The figure shows three views and two pictorial views of one solid part (mm, origin at its lowest corner). Answer the questions. Give positions to 0.01 mm unless a question says otherwise; leave off trailing zeros. Write each loop counter-clockwise with the first axis right and the second up, starting at its lowest first coordinate (ties: lowest second). Pieces come first, ordered by that corner, then holes. Notation, with made-up numbers: (-3.5, 88.5) -> (26.5, 88.5) arc R17 cw to (26.5, 101.5) -> close; hole circle Ø2 at (-24.5, 12.5). An arc over 180 degrees is marked (long way). Write each question's results on one line, items separated by ' | '. Start each with the question number.
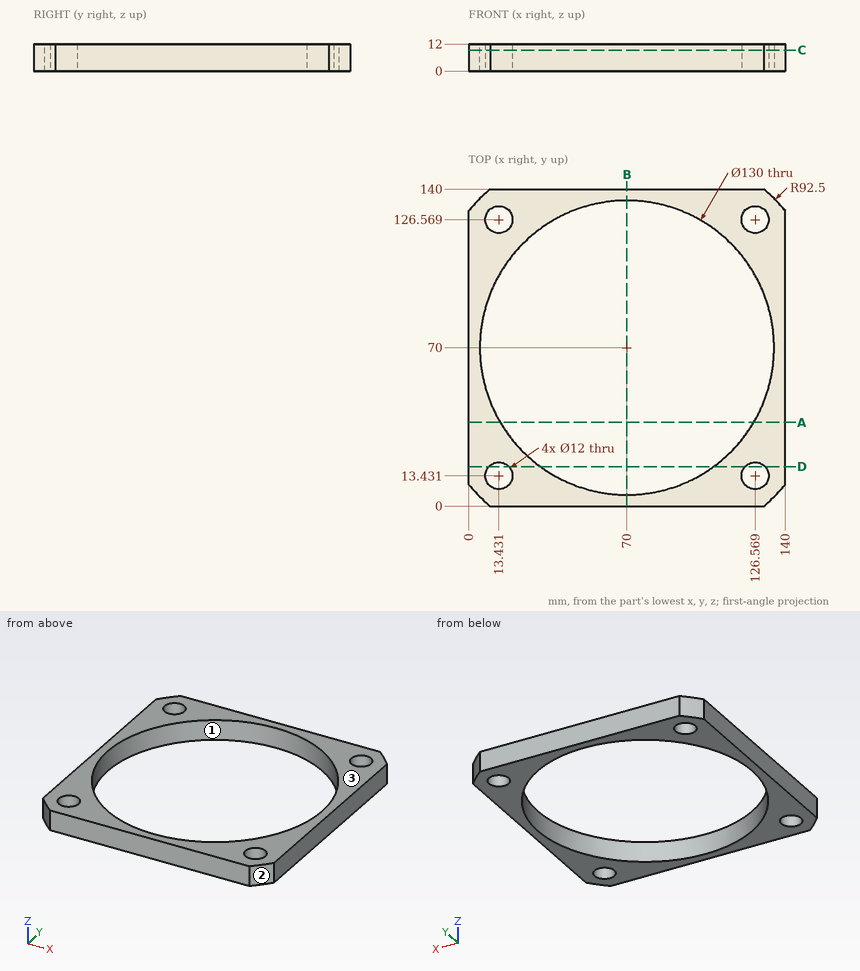
1. Section D-D (y = 17.5) is taken. Write down the section's boundary in (x, z) (1 decimal).
2. Section C-C (z = 9.25) is taken. Write down the section's boundary in (x, y).
3. Consider probe 1 along Y at (x, z) = (70, 2.5); probe 2 along X at (y, z) = (16, 2.75) (1 decimal); probe 3 along X at (y, z) = (18.5, 0.75) (1 decimal). Determine where each line is inside the solid, lowest interval first. Write a range as [from, to].
4. Section B-B (x = 70) is taken. Write down the section's boundary in (y, z), then the cut area to 3 significant figures.
5. Each of these flat-tipped pins is pushed along its axis until it touches: pin 1 Ø7 at (x, y) = (126.57, 13.43) entering from -Z; pin 2 Ø15.5 at (x, y) = (13.43, 13.43) entering from +Z. Where does it stop, or does it pass through?
6. The mould has two halves that part along Y. Classify the marked faces 1, 2 and 3: pulls with the +Y half, pulls with the -Y half, needs draft (parallel to the pull), parting line crosses it, or undercut.
7. Section A-A (y = 37) is taken. Write down the section's boundary in (x, z).
Results:
1) outline: (0, 0) -> (9, 0) -> (9, 12) -> (0, 12) -> close; (17.8, 0) -> (31.7, 0) -> (31.7, 12) -> (17.8, 12) -> close; (108.3, 0) -> (122.2, 0) -> (122.2, 12) -> (108.3, 12) -> close; (131, 0) -> (140, 0) -> (140, 12) -> (131, 12) -> close
2) outline: (0, 9.53) arc R92.5 ccw to (9.53, 0) -> (130.47, 0) arc R92.5 ccw to (140, 9.53) -> (140, 130.47) arc R92.5 ccw to (130.47, 140) -> (9.53, 140) arc R92.5 ccw to (0, 130.47) -> close; hole circle Ø130 at (70, 70); hole circle Ø12 at (13.43, 13.43); hole circle Ø12 at (13.43, 126.57); hole circle Ø12 at (126.57, 13.43); hole circle Ø12 at (126.57, 126.57)
3) probe 1: y = [0, 5], [135, 140] | probe 2: x = [0, 8], [18.9, 33.8], [106.2, 121.1], [132, 140] | probe 3: x = [0, 10.2], [16.6, 30.3], [109.7, 123.4], [129.8, 140]
4) outline: (0, 0) -> (5, 0) -> (5, 12) -> (0, 12) -> close; (135, 0) -> (140, 0) -> (140, 12) -> (135, 12) -> close | area: 120 mm²
5) pin 1: passes through | pin 2: stops at z = 12
6) face 1: undercut | face 2: pulls with the -Y half | face 3: needs draft
7) outline: (0, 0) -> (14, 0) -> (14, 12) -> (0, 12) -> close; (126, 0) -> (140, 0) -> (140, 12) -> (126, 12) -> close
